For this review, take the finished solid that the model builds, in its own axes (mm). A direction names the side the tool comes from. Coordinates: 2 decimals unless noted, no trailing zeros. One line per item, written item: value. Start each with the question number.
1. Take a section at A-A, the plane z = -22. Count the separate pieces of the cut face and the enclosed holes in it, and give its area (3 significant figures).
2. To check wall thickness, follow line 1 (Y direction, x = -2.5, z = -50.5); line 2 (Y direction, x = -9, z = -64.5); line 3 (Y direction, x = 7.75, z = -119). State the ranges of each line that lie inside material, in increasing order. Write a range as from..to.
3. The part is to be moulded in two halves that separate along Y. For faces 1 (the face through (6, 30, -148)), 2 (the face through (10, -10, -148)), 3 (the face through (0, 4, -148)), say which applies: released by +Y, released by -Y, zero draft, split by the parting line, or undercut.
4. For faces 4 (the face through (0, -4, -148)), 5 (the face through (6, -30, -148)), list the 3-axis set-ups (+Z, -Z, +X, -X, +Y, -Y) from which the entire face can be reached by the end or side of a thin tool; tool diameter is ignored.
5. Insertion check: pin 1 (1 mm diameter, centred on x = 1.5, z = -191.5, fed in from +Y); pin 2 (0.7 mm diameter, centred on y = -18.5, z = -165, fed in from -X). Each pin has a flat end and moves straight along its axis. Give the tip position at first contact, or say it passes through.
```python
from build123d import *

# Parameters (mm, degrees)
SKETCH1_R           = 2.0999999
BOSS_EXTRUDE1_DEPTH = 300


with BuildPart() as part:
    # Sketch1 → Boss-Extrude1 (new body)
    with BuildSketch(Plane.XY):
        with BuildLine():
            Line((-10, 16.7), (-10, 3.3))
            ThreePointArc((-10, 3.3), (-9.912132034, 3.087867966), (-9.7, 3))
            Line((-9.7, 3), (-8, 3))
            Line((-8, 3), (-8, 6))
            Line((-8, 6), (-7.060650687, 6))
            Line((-7.060650687, 6), (-4, 2.939349))
            Line((-4, 2.939349), (-4, 0.519615242))
            Line((-4, 0.519615242), (-3.7, 0))
            Line((-3.7, 0), (-4, -0.519615242))
            Line((-4, -0.519615242), (-4, -2.9393502))
            Line((-4, -2.9393502), (-7.060649487, -6))
            Line((-7.060649487, -6), (-8, -6))
            Line((-8, -6), (-8, -3))
            Line((-8, -3), (-9.7, -3))
            ThreePointArc((-9.7, -3), (-9.912132034, -3.087867966), (-10, -3.3))
            Line((-10, -3.3), (-10, -16.7))
            ThreePointArc((-10, -16.7), (-9.912132034, -16.912132034), (-9.7, -17))
            Line((-9.7, -17), (-8, -17))
            Line((-8, -17), (-8, -14))
            Line((-8, -14), (-7.060672887, -14))
            Line((-7.060672887, -14), (-4, -17.0606732))
            Line((-4, -17.0606732), (-4, -19.480384758))
            Line((-4, -19.480384758), (-3.7, -20))
            Line((-3.7, -20), (-4, -20.519615242))
            Line((-4, -20.519615242), (-4, -22.93935665))
            Line((-4, -22.93935665), (-7.060643037, -26))
            Line((-7.060643037, -26), (-8, -26))
            Line((-8, -26), (-8, -23))
            Line((-8, -23), (-9.7, -23))
            ThreePointArc((-9.7, -23), (-9.912132034, -23.087867966), (-10, -23.3))
            Line((-10, -23.3), (-10, -29))
            ThreePointArc((-10, -29), (-9.707106781, -29.707106781), (-9, -30))
            Line((-9, -30), (-3.3, -30))
            ThreePointArc((-3.3, -30), (-3.087867966, -29.912132034), (-3, -29.7))
            Line((-3, -29.7), (-3, -28))
            Line((-3, -28), (-6, -28))
            Line((-6, -28), (-6, -27.060683408))
            Line((-6, -27.060683408), (-2.939316, -24))
            Line((-2.939316, -24), (-0.519095055, -24))
            Line((-0.519095055, -24), (1e-06, -23.7))
            Line((1e-06, -23.7), (0.518577868, -24))
            Line((0.518577868, -24), (2.939318, -24))
            Line((2.939318, -24), (6, -27.060682403))
            Line((6, -27.060682403), (6, -28))
            Line((6, -28), (3, -28))
            Line((3, -28), (3, -29.7))
            ThreePointArc((3, -29.7), (3.087867966, -29.912132034), (3.3, -30))
            Line((3.3, -30), (9, -30))
            ThreePointArc((9, -30), (9.707106781, -29.707106781), (10, -29))
            Line((10, -29), (10, -23.3))
            ThreePointArc((10, -23.3), (9.912132034, -23.087867966), (9.7, -23))
            Line((9.7, -23), (8, -23))
            Line((8, -23), (8, -26))
            Line((8, -26), (7.060637687, -26))
            Line((7.060637687, -26), (4, -22.93935641))
            Line((4, -22.93935641), (4, -20.519623992))
            Line((4, -20.519623992), (3.7, -20.00000875))
            Line((3.7, -20.00000875), (4, -19.480393508))
            Line((4, -19.480393508), (4, -17.06066109))
            Line((4, -17.06066109), (7.060655187, -14))
            Line((7.060655187, -14), (8, -14))
            Line((8, -14), (8, -17))
            Line((8, -17), (9.7, -17))
            ThreePointArc((9.7, -17), (9.912132034, -16.912132034), (10, -16.7))
            Line((10, -16.7), (10, -3.3))
            ThreePointArc((10, -3.3), (9.912132034, -3.087867966), (9.7, -3))
            Line((9.7, -3), (8, -3))
            Line((8, -3), (8, -6))
            Line((8, -6), (7.060651537, -6))
            Line((7.060651537, -6), (4, -2.93934815))
            Line((4, -2.93934815), (4, -0.519623992))
            Line((4, -0.519623992), (3.7, -8.75e-06))
            Line((3.7, -8.75e-06), (4, 0.519606492))
            Line((4, 0.519606492), (4, 2.9393426))
            Line((4, 2.9393426), (7.060657087, 6))
            Line((7.060657087, 6), (8, 6))
            Line((8, 6), (8, 3))
            Line((8, 3), (9.7, 3))
            ThreePointArc((9.7, 3), (9.912132034, 3.087867966), (10, 3.3))
            Line((10, 3.3), (10, 16.7))
            ThreePointArc((10, 16.7), (9.912132034, 16.912132034), (9.7, 17))
            Line((9.7, 17), (8, 17))
            Line((8, 17), (8, 14))
            Line((8, 14), (7.06065821, 14))
            Line((7.06065821, 14), (4, 17.060658523))
            Line((4, 17.060658523), (4, 19.480376008))
            Line((4, 19.480376008), (3.7, 19.99999125))
            Line((3.7, 19.99999125), (4, 20.519606492))
            Line((4, 20.519606492), (4, 22.939362173))
            Line((4, 22.939362173), (7.060637514, 26))
            Line((7.060637514, 26), (8, 26))
            Line((8, 26), (8, 23))
            Line((8, 23), (9.7, 23))
            ThreePointArc((9.7, 23), (9.912132034, 23.087867966), (10, 23.3))
            Line((10, 23.3), (10, 29))
            ThreePointArc((10, 29), (9.707106781, 29.707106781), (9, 30))
            Line((9, 30), (3.3, 30))
            ThreePointArc((3.3, 30), (3.087867966, 29.912132034), (3, 29.7))
            Line((3, 29.7), (3, 28))
            Line((3, 28), (6, 28))
            Line((6, 28), (6, 27.060684313))
            Line((6, 27.060684313), (2.939316, 24))
            Line((2.939316, 24), (0.519614242, 24))
            Line((0.519614242, 24), (-1e-06, 23.7))
            Line((-1e-06, 23.7), (-0.519616242, 24))
            Line((-0.519616242, 24), (-2.939318, 24))
            Line((-2.939318, 24), (-6, 27.060682313))
            Line((-6, 27.060682313), (-6, 28))
            Line((-6, 28), (-3, 28))
            Line((-3, 28), (-3, 29.7))
            ThreePointArc((-3, 29.7), (-3.087867966, 29.912132034), (-3.3, 30))
            Line((-3.3, 30), (-9, 30))
            ThreePointArc((-9, 30), (-9.707106781, 29.707106781), (-10, 29))
            Line((-10, 29), (-10, 23.3))
            ThreePointArc((-10, 23.3), (-9.912132034, 23.087867966), (-9.7, 23))
            Line((-9.7, 23), (-8, 23))
            Line((-8, 23), (-8, 26))
            Line((-8, 26), (-7.060644014, 26))
            Line((-7.060644014, 26), (-4, 22.939355673))
            Line((-4, 22.939355673), (-4, 20.519615242))
            Line((-4, 20.519615242), (-3.7, 20))
            Line((-3.7, 20), (-4, 19.480384758))
            Line((-4, 19.480384758), (-4, 17.060669373))
            Line((-4, 17.060669373), (-7.06066906, 14))
            Line((-7.06066906, 14), (-8, 14))
            Line((-8, 14), (-8, 17))
            Line((-8, 17), (-9.7, 17))
            ThreePointArc((-9.7, 17), (-9.912132034, 16.912132034), (-10, 16.7))
        make_face()
        with Locations((0, 20.000013123)):
            Circle(SKETCH1_R, mode=Mode.SUBTRACT)
        Circle(SKETCH1_R, mode=Mode.SUBTRACT)
        with Locations((0, -20.000013525)):
            Circle(SKETCH1_R, mode=Mode.SUBTRACT)
        with BuildLine():
            Line((-7.7, 8), (-7.063594325, 8))
            ThreePointArc((-7.063594325, 8), (-6.948789288, 7.977163857), (-6.85146228, 7.912132024))
            Line((-6.85146228, 7.912132024), (-2.939330656, 4))
            Line((-2.939330656, 4), (2.939337056, 4))
            Line((2.939337056, 4), (6.85146868, 7.912132024))
            ThreePointArc((6.85146868, 7.912132024), (6.948795688, 7.977163857), (7.063600725, 8))
            Line((7.063600725, 8), (7.7, 8))
            ThreePointArc((7.7, 8), (7.912132034, 8.087867966), (8, 8.3))
            Line((8, 8.3), (8, 11.7))
            ThreePointArc((8, 11.7), (7.912132034, 11.912132034), (7.7, 12))
            Line((7.7, 12), (7.063601848, 12))
            ThreePointArc((7.063601848, 12), (6.948796811, 12.022836143), (6.851469803, 12.087867976))
            Line((6.851469803, 12.087867976), (2.939338179, 16))
            Line((2.939338179, 16), (-2.939349029, 16))
            Line((-2.939349029, 16), (-6.851480653, 12.087867976))
            ThreePointArc((-6.851480653, 12.087867976), (-6.948807661, 12.022836143), (-7.063612698, 12))
            Line((-7.063612698, 12), (-7.7, 12))
            ThreePointArc((-7.7, 12), (-7.912132034, 11.912132034), (-8, 11.7))
            Line((-8, 11.7), (-8, 8.3))
            ThreePointArc((-8, 8.3), (-7.912132034, 8.087867966), (-7.7, 8))
        make_face(mode=Mode.SUBTRACT)
        with BuildLine():
            Line((-8, -8.3), (-8, -11.7))
            ThreePointArc((-8, -11.7), (-7.912132034, -11.912132034), (-7.7, -12))
            Line((-7.7, -12), (-7.063616525, -12))
            ThreePointArc((-7.063616525, -12), (-6.948811488, -12.022836143), (-6.85148448, -12.087867976))
            Line((-6.85148448, -12.087867976), (-2.939352856, -16))
            Line((-2.939352856, -16), (2.939340746, -16))
            Line((2.939340746, -16), (6.851465031, -12.08786817))
            ThreePointArc((6.851465031, -12.08786817), (6.948792107, -12.022836196), (7.06359727, -12))
            Line((7.06359727, -12), (7.7, -12))
            ThreePointArc((7.7, -12), (7.912132034, -11.912132034), (8, -11.7))
            Line((8, -11.7), (8, -8.3))
            ThreePointArc((8, -8.3), (7.912132034, -8.087867966), (7.7, -8))
            Line((7.7, -8), (7.063595175, -8))
            ThreePointArc((7.063595175, -8), (6.948790138, -7.977163857), (6.85146313, -7.912132024))
            Line((6.85146313, -7.912132024), (2.939331506, -4))
            Line((2.939331506, -4), (-2.939329456, -4))
            Line((-2.939329456, -4), (-6.85146108, -7.912132024))
            ThreePointArc((-6.85146108, -7.912132024), (-6.948788088, -7.977163857), (-7.063593125, -8))
            Line((-7.063593125, -8), (-7.7, -8))
            ThreePointArc((-7.7, -8), (-7.912132034, -8.087867966), (-8, -8.3))
        make_face(mode=Mode.SUBTRACT)
    extrude(amount=-BOSS_EXTRUDE1_DEPTH)


solid = part.part
```
Solutions:
1. separate pieces: 1
1. enclosed holes: 5
1. area: 465 mm2
2. line 1: -24..-16, -4..4, 16..24
2. line 2: -30..-23, -17..-3, 3..17, 23..30
2. line 3: -30..-26, -14..-12, -8..-6, 6..8, 12..14, 26..30
3. face 1: released by +Y
3. face 2: zero draft
3. face 3: undercut
4. face 4: +Z, -Z
4. face 5: +Z, -Z, +X, -X, -Y
5. pin 1: y = 24
5. pin 2: x = -4
